Read the model definition and answer for the solid it produces. Units are mm, in the model's axes. A direction names the side the tool comes from. Round coordinates to 2 decimals unless told otherwise and drop trailing zeros. Order: outer loops, then holes, each group sorted by start corner. A loop starts at its lowest first (then second) coordinate and runs counter-clockwise, first axis right, second up. Notation, with made-up numbers: (2.5, 45) -> (38.5, 45) arc R23 ccw to (38.5, 55) -> close; hole circle Ø9 at (-18.5, 53.25). An arc over 180 degrees is marked (long way). Use a Markdown table: item, result. Add a question column.
1. Section C-C, the plane x = -32.5 is taken. Give the vertices of the cut face in (y, z).
2. For faces 1 (the face through (-36.923, -26, 28)), 2 (the face through (-36.923, -26, 20)), 3 (the face through (-22.923, -25.9, 24)), determine the directions among +Z, -Z, +X, -X, +Y, -Y from which every point of the face is accessible in a straight line to the end or side of a thin tool.
3. Section B-B, the plane y = -4 is taken. Give the vertices of the cut face in (x, z).
4. Consider L1, parallel to Z at x = -28.25, y = -4.5; L2, parallel to Z at x = -34.75, y = -5.5; L3, parallel to X at y = -29, z = 24.5. Determine where each line is inside the solid, lowest interval first. Write a range as [from, to].
5. The mould has two halves that part along Z. Classify faces 4 (the face through (-39.923, -11, 28)), 5 (the face through (-31.41, -4.06, 31.56)), 6 (the face through (-29, -11, 28.942)): +Z half, -Z half, draft (parallel to the pull), parting line (faces both ways), or undercut.
6. Given pin 1 (6.5 mm diameter, centred on x = -32.92, z = 12.94, fed in from -Y); pin 2 (2 mm diameter, centred on x = -21.5, y = -15, fed in from +Z); pin 3 (2 mm diameter, centred on x = -24.5, z = 22.5, fed in from -Y); pin 4 (5.5 mm diameter, centred on x = -28.5, y = -18, fed in from +Z), each flat-ended and moving along its own axis, determine where each tip first touches the part or whether it passes through.
7. Section D-D, the plane z = 31.5 is taken. Give the vertices of the cut face in (x, y), then the cut area to 3 significant figures.
8. Section A-A, the plane y = -23.5 is taken. Give the vertices of the cut face in (x, z).
```python
from build123d import *

# Parameters (mm, degrees)
F0_W     = 22
F0_H     = 42
F1_DEPTH = 3
F2_W     = 3
F2_H     = 30
F2_W_2   = 5
F3_DEPTH = 22
F4_D     = 4.1
F7_DEPTH = 5
F8_DEPTH = 2.97
F9_R     = 4.99999
F11_D    = 4.1
F12_D    = 2.8


# Not quite as in the source:
# - a fillet or chamfer is up to 0.001 mm smaller than in the source, because OpenCascade refuses the exact size


with BuildPart() as f1:
    # F0 (on Front) → F1 (new body)
    with BuildSketch(Plane.XZ):
        with Locations((-28.9233987555, 27.9422005266)):
            Rectangle(F0_W, F0_H)
    extrude(amount=F1_DEPTH)

    # F2 (on face) → F3 (join)
    with BuildSketch(Plane(origin=(-39.9233987555, 0, 0), x_dir=(0, -1, 0), z_dir=(-1, 0, 0))):
        with Locations((1.5, 33.9422005266)):
            Rectangle(F2_W, F2_H)
        with Locations((5.5, 33.9422005266)):
            Rectangle(F2_W_2, F2_H)
    extrude(amount=-F3_DEPTH)

    # F4 (through all)
    with Locations(Plane(origin=(0, 0, 0), x_dir=(1, 0, 0), z_dir=(0, 1, 0))):
        with Locations((-24.9233987555, -12.9422005266), (-32.9233987555, -12.9422005266), (-32.9233987555, -32.9422005266), (-24.9233987555, -32.9422005266)):
            Hole(F4_D / 2)

    # F6 (on line) → F7 (join, symmetric)
    with BuildSketch(Plane.XY.offset(23.9422005266)):
        with BuildLine():
            ThreePointArc((-36.9233987555, -20), (-28.9233987555, -12), (-20.9233987555, -20))
            Line((-20.9233987555, -20), (-20.9233987555, -32))
            Line((-20.9233987555, -32), (-17.9233987555, -32))
            Line((-17.9233987555, -32), (-17.9233987555, 0))
            Line((-17.9233987555, 0), (-39.9233987555, 0))
            Line((-39.9233987555, 0), (-39.9233987555, -32))
            Line((-39.9233987555, -32), (-36.9233987555, -32))
            Line((-36.9233987555, -32), (-36.9233987555, -20))
        make_face()
    extrude(amount=F7_DEPTH, both=True)

    # F6 (on line) → F8 (join, symmetric)
    with BuildSketch(Plane.XY.offset(23.9422005266)):
        with BuildLine():
            ThreePointArc((-34.9233987555, -20), (-28.9233987555, -14), (-22.9233987555, -20))
            Line((-22.9233987555, -20), (-22.9233987555, -25.2915026221))
            ThreePointArc((-22.9233987555, -25.2915026221), (-21.4400839819, -22.8284271247), (-20.9233987555, -20))
            ThreePointArc((-20.9233987555, -20), (-28.9233987555, -12), (-36.9233987555, -20))
            ThreePointArc((-36.9233987555, -20), (-36.406713529, -22.8284271247), (-34.9233987555, -25.2915026221))
            Line((-34.9233987555, -25.2915026221), (-34.9233987555, -20))
        make_face()
        with BuildLine():
            Line((-34.9233987555, -32), (-34.9233987555, -25.2915026221))
            ThreePointArc((-34.9233987555, -25.2915026221), (-36.406713529, -22.8284271247), (-36.9233987555, -20))
            Line((-36.9233987555, -20), (-36.9233987555, -32))
            Line((-36.9233987555, -32), (-34.9233987555, -32))
        make_face()
        with BuildLine():
            ThreePointArc((-20.9233987555, -20), (-21.4400839819, -22.8284271247), (-22.9233987555, -25.2915026221))
            Line((-22.9233987555, -25.2915026221), (-22.9233987555, -32))
            Line((-22.9233987555, -32), (-20.9233987555, -32))
            Line((-20.9233987555, -32), (-20.9233987555, -20))
        make_face()
    extrude(amount=F8_DEPTH, both=True)

    # F9 (radius 5 in the source; OpenCascade refuses exactly that, so slightly less here)
    f9_edges = [f1.edges().sort_by_distance(p)[0] for p in [
        (-38.423399, -32, 28.942201),
        (-38.423399, -32, 18.942201),
        (-19.423399, -32, 18.942201),
        (-19.423399, -32, 28.942201),
    ]]
    fillet(f9_edges, radius=F9_R)

    # F11 (through all)
    with Locations(Plane(origin=(-39.9233987555, 0, 0), x_dir=(0, -1, 0), z_dir=(-1, 0, 0))):
        with Locations((4, 44.9422005266), (4, 24.9422005266)):
            Hole(F11_D / 2)

    # F12 (through all)
    with Locations(Plane(origin=(-39.9233987555, 0, 0), x_dir=(0, -1, 0), z_dir=(-1, 0, 0))):
        with Locations((27.5, 23.9422005266)):
            Hole(F12_D / 2)


solid = f1.part
```
Verdict:
| question | item | result |
|---|---|---|
| 1 | outline | (-15.18, 20.97) -> (-12.84, 20.97) -> (-12.84, 18.94) -> (-3, 18.94) -> (-3, 14.95) -> (0, 14.95) -> (0, 30.94) -> (-8, 30.94) -> (-8, 28.94) -> (-12.84, 28.94) -> (-12.84, 26.91) -> (-15.18, 26.91) -> close; (-8, 34.95) -> (0, 34.95) -> (0, 48.94) -> (-8, 48.94) -> close; (-3, 6.94) -> (0, 6.94) -> (0, 10.94) -> (-3, 10.94) -> close; hole circle Ø4.1 at (-4, 24.94); hole circle Ø4.1 at (-4, 44.94) |
| 2 | face 1 | +Z, -Y |
| 2 | face 2 | -Z, -Y |
| 2 | face 3 | +Z, -Z, -Y |
| 3 | outline | (-39.92, 18.94) -> (-17.92, 18.94) -> (-17.92, 22.89) -> (-39.92, 22.89) -> close; (-39.92, 26.99) -> (-17.92, 26.99) -> (-17.92, 42.89) -> (-39.92, 42.89) -> close; (-39.92, 46.99) -> (-17.92, 46.99) -> (-17.92, 48.94) -> (-39.92, 48.94) -> close; hole circle Ø4.1 at (-32.92, 32.94); hole circle Ø4.1 at (-24.92, 32.94) |
| 4 | L1 | z = [18.94, 22.95], [26.93, 42.95], [46.93, 48.94] |
| 4 | L2 | z = [18.94, 23.54], [26.34, 32.01], [33.87, 43.54], [46.34, 48.94] |
| 4 | L3 | x = [-39.92, -34.92], [-22.92, -17.92] |
| 5 | face 4 | draft |
| 5 | face 5 | undercut |
| 5 | face 6 | +Z half |
| 6 | pin 1 | stops at y = -3 |
| 6 | pin 2 | stops at z = 28.94 |
| 6 | pin 3 | stops at y = -17.43 |
| 6 | pin 4 | passes through |
| 7 | outline | (-39.92, -8) -> (-34.38, -8) -> (-34.38, 0) -> (-39.92, 0) -> close; (-31.47, -8) -> (-26.38, -8) -> (-26.38, 0) -> (-31.47, 0) -> close; (-23.47, -8) -> (-17.92, -8) -> (-17.92, 0) -> (-23.47, 0) -> close |
| 7 | area | 129 mm2 |
| 8 | outline | (-39.92, 18.94) -> (-36.92, 18.94) -> (-36.92, 20.97) -> (-34.92, 20.97) -> (-34.92, 26.91) -> (-36.92, 26.91) -> (-36.92, 28.94) -> (-39.92, 28.94) -> close; (-22.92, 20.97) -> (-20.92, 20.97) -> (-20.92, 18.94) -> (-17.92, 18.94) -> (-17.92, 28.94) -> (-20.92, 28.94) -> (-20.92, 26.91) -> (-22.92, 26.91) -> close |
